Here's how the part is built. I have some questions about the finished solid (model axes, mm). A direction names the side the tool comes from. Round coordinates to 2 decimals unless told otherwise and drop trailing zeros. Order: outer loops, then holes, each group sorted by start corner. A loop starts at its lowest first (then second) coordinate and runs counter-clockwise, first axis right, second up.
```python
from build123d import *

# Parameters (mm, degrees)
BOX_W           = 21
BOX_H           = 32
BOX_DEPTH       = 5
SKETCH_R        = 5.5
POCKET_DEPTH    = 5.001
SKETCH001_R     = 1.5
POCKET001_DEPTH = 5.001
SKETCH002_W     = 21
SKETCH002_H     = 2
POCKET002_DEPTH = 2


with BuildPart() as part:
    # Box → Box (new body)
    with BuildSketch(Plane.XY):
        with Locations((10.5, 16)):
            Rectangle(BOX_W, BOX_H)
    extrude(amount=BOX_DEPTH)

    # Sketch → Pocket (cut, through all)
    with BuildSketch(Plane.XY.offset(5)):
        with Locations((10.5, 16)):
            Circle(SKETCH_R)
    extrude(amount=-POCKET_DEPTH, mode=Mode.SUBTRACT)

    # Sketch001 → Pocket001 (cut, through all)
    with BuildSketch(Plane.XY.offset(5)):
        with Locations((5, 27)):
            Circle(SKETCH001_R)
        with Locations((16, 27)):
            Circle(SKETCH001_R)
        with Locations((5, 5)):
            Circle(SKETCH001_R)
        with Locations((16, 5)):
            Circle(SKETCH001_R)
    extrude(amount=-POCKET001_DEPTH, mode=Mode.SUBTRACT)

    # Sketch002 → Pocket002 (cut)
    with BuildSketch(Plane.XY.offset(5)):
        with Locations((10.5, 1)):
            Rectangle(SKETCH002_W, SKETCH002_H)
        with Locations((10.5, 31)):
            Rectangle(SKETCH002_W, SKETCH002_H)
    extrude(amount=-POCKET002_DEPTH, mode=Mode.SUBTRACT)


solid = part.part
```
1) We'd pull the mould along X, two halves only. Please class faces 4 (the cylindrical face through (14.5, 5.07, 2.54)), 5 (the flat face through (21, 16, 2)), 6 (the flat face through (0, 16, 2)), 7 (the flat face through (5.7, 19.3, 5)): +X half, -X half, draft (parallel to the pull), parting line (faces both ways), or undercut.
2) If we section it at B-B (z = 1.1): Write out the boundary of the cut face in (x, y), plus the area to 3 significant figures.
3) For faces 1 (the flat face through (10, 2, 4)), 2 (the flat face through (10, 0, 1)), 3 (the flat face through (10, 31, 3)), which set-ups out of +Z, -Z, +X, -X, +Y, -Y let a thin tool reach every point of the face, with its end or its side?
4) I'm going to push flat-ended pins straight in: pin 1 (2.5 mm diameter, centred on x = 16, y = 27, fed in from -Z); pin 2 (1.6 mm diameter, centred on x = 9, y = 1, fed in from +Z); pin 3 (1.6 mm diameter, centred on x = 13.5, z = 4.5, fed in from -Y); pin 4 (0.6 mm diameter, centred on x = 15, z = 4.5, fed in from +Y). Where does each tip first touch, or does it pass through?
5) If we section it at A-A (x = 10.5): Write out the boundary of the cut face in (y, z), plus the area to 3 significant figures.
6) If we section it at C-C (y = 16): Write out the boundary of the cut face in (x, z).
7) If we section it at D-D (y = 4): Write out the boundary of the cut face in (x, z), plus the area to 3 significant figures.
8) I need wall thicknesses on line 1 (X direction, y = 4, z = 1.6); line 2 (X direction, y = 27.5, z = 3.6); line 3 (Y direction, x = 6.75, z = 1.9). Which ranges of each line are inside material? Lowest first, please.
Solutions:
1. face 4: undercut
1. face 5: +X half
1. face 6: -X half
1. face 7: draft
2. outline: (0, 0) - (21, 0) - (21, 32) - (0, 32) - close; hole circle Ø3 at (5, 5); hole circle Ø3 at (5, 27); hole circle Ø11 at (10.5, 16); hole circle Ø3 at (16, 5); hole circle Ø3 at (16, 27)
2. area: 549 mm2
3. face 1: +Z, +X, -X, -Y
3. face 2: +Z, -Z, +X, -X, -Y
3. face 3: +Z, +X, -X, +Y
4. pin 1: passes through
4. pin 2: stops at z = 3
4. pin 3: stops at y = 2
4. pin 4: stops at y = 30
5. outline: (0, 0) - (10.5, 0) - (10.5, 5) - (2, 5) - (2, 3) - (0, 3) - close; (21.5, 0) - (32, 0) - (32, 3) - (30, 3) - (30, 5) - (21.5, 5) - close
5. area: 97.0 mm2
6. outline: (0, 0) - (5, 0) - (5, 5) - (0, 5) - close; (16, 0) - (21, 0) - (21, 5) - (16, 5) - close
7. outline: (0, 0) - (3.88, 0) - (3.88, 5) - (0, 5) - close; (6.12, 0) - (14.88, 0) - (14.88, 5) - (6.12, 5) - close; (17.12, 0) - (21, 0) - (21, 5) - (17.12, 5) - close
7. area: 82.6 mm2
8. line 1: x = 0 to 3.88, 6.12 to 14.88, 17.12 to 21
8. line 2: x = 0 to 3.59, 6.41 to 14.59, 17.41 to 21
8. line 3: y = 0 to 11.98, 20.02 to 32
